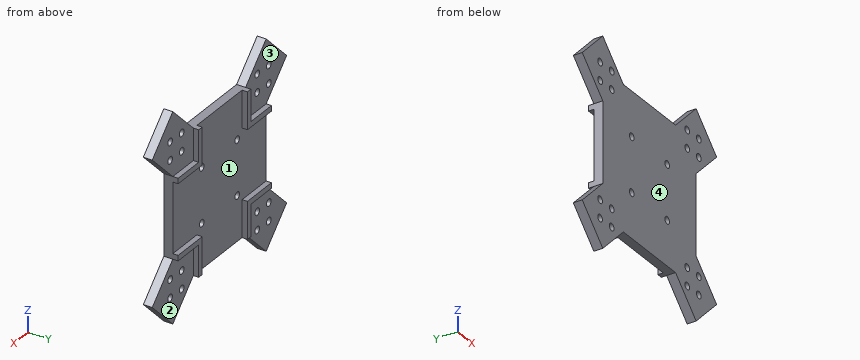
from build123d import *

# Parameters (mm, degrees)
EXTRUDE_1_DEPTH     = 5
EXTRUDE_2_DEPTH     = 3
SKETCH_4_R          = 2
CUT_EXTRUDE_1_DEPTH = 5
SKETCH_6_R          = 2
CUT_EXTRUDE_2_DEPTH = 5


with BuildPart() as part:
    # 스케치1 → 보스-돌출1 (new body)
    with BuildSketch(Plane(origin=(0, 0, 0), x_dir=(1, 0, 0), z_dir=(0, 1, 0))):
        Polygon((-40.17766953, 22.5), (-57.855339059, 40.17766953), (-40.17766953, 57.855339059), (-22.5, 40.17766953), align=None)
        Polygon((-22.5, 40.17766953), (22.5, -40.17766953), (-22.5, -40.17766953), (-40.17766953, -22.5), (-40.17766953, 22.5), align=None)
        Polygon((-40.17766953, -57.855339059), (-57.855339059, -40.17766953), (-40.17766953, -22.5), (-22.5, -40.17766953), align=None)
        Polygon((-22.5, 40.17766953), (22.5, 40.17766953), (40.17766953, 22.5), (40.17766953, -22.5), (22.5, -40.17766953), align=None)
        Polygon((40.17766953, -57.855339059), (22.5, -40.17766953), (40.17766953, -22.5), (57.855339059, -40.17766953), align=None)
        Polygon((40.17766953, 22.5), (22.5, 40.17766953), (40.17766953, 57.855339059), (57.855339059, 40.17766953), align=None)
    extrude(amount=EXTRUDE_1_DEPTH)

    # 스케치2 → 보스-돌출2 (add)
    with BuildSketch(Plane(origin=(0, 5, 0), x_dir=(1, 0, 0), z_dir=(0, 1, 0))):
        Polygon((-40.17766953, -19.5), (-40.17766953, -22.5), (-22.5, -22.5), (-22.5, -40.17766953), (-19.5, -40.17766953), (-19.5, -19.5), align=None)
        Polygon((-19.5, 40.17766953), (-22.5, 40.17766953), (-22.5, 22.5), (-40.17766953, 22.5), (-40.17766953, 19.5), (-19.5, 19.5), align=None)
        Polygon((40.17766953, 19.5), (40.17766953, 22.5), (22.5, 22.5), (22.5, 40.17766953), (19.5, 40.17766953), (19.5, 19.5), align=None)
        Polygon((19.5, -40.17766953), (22.5, -40.17766953), (22.5, -22.5), (40.17766953, -22.5), (40.17766953, -19.5), (19.5, -19.5), align=None)
    extrude(amount=EXTRUDE_2_DEPTH)

    # 스케치4 → 컷-돌출1 (cut)
    with BuildSketch(Plane(origin=(0, 0, 0), x_dir=(1, 0, 0), z_dir=(0, 1, 0))):
        with Locations(Location((-42.5, -42.5, 0), (0, 0, 270))):
            Circle(SKETCH_4_R)
        with Locations(Location((-32.5, -42.5, 0), (0, 0, 270))):
            Circle(SKETCH_4_R)
        with Locations(Location((-42.5, -32.5, 0), (0, 0, 270))):
            Circle(SKETCH_4_R)
        with Locations(Location((-32.5, -32.5, 0), (0, 0, 270))):
            Circle(SKETCH_4_R)
        with Locations(Location((-32.5, 32.5, 0), (0, 0, 270))):
            Circle(SKETCH_4_R)
        with Locations(Location((-42.5, 32.5, 0), (0, 0, 270))):
            Circle(SKETCH_4_R)
        with Locations(Location((-42.5, 42.5, 0), (0, 0, 270))):
            Circle(SKETCH_4_R)
        with Locations(Location((-32.5, 42.5, 0), (0, 0, 270))):
            Circle(SKETCH_4_R)
        with Locations(Location((32.5, 32.5, 0), (0, 0, 270))):
            Circle(SKETCH_4_R)
        with Locations(Location((32.5, 42.5, 0), (0, 0, 270))):
            Circle(SKETCH_4_R)
        with Locations(Location((42.5, 42.5, 0), (0, 0, 270))):
            Circle(SKETCH_4_R)
        with Locations(Location((42.5, 32.5, 0), (0, 0, 270))):
            Circle(SKETCH_4_R)
        with Locations(Location((32.5, -32.5, 0), (0, 0, 270))):
            Circle(SKETCH_4_R)
        with Locations(Location((42.5, -32.5, 0), (0, 0, 270))):
            Circle(SKETCH_4_R)
        with Locations(Location((42.5, -42.5, 0), (0, 0, 270))):
            Circle(SKETCH_4_R)
        with Locations(Location((32.5, -42.5, 0), (0, 0, 270))):
            Circle(SKETCH_4_R)
    extrude(amount=CUT_EXTRUDE_1_DEPTH, mode=Mode.SUBTRACT)

    # 스케치6 → 컷-돌출2 (cut)
    with BuildSketch(Plane(origin=(0, 0, 0), x_dir=(1, 0, 0), z_dir=(0, 1, 0))):
        with Locations(Location((-15.25, 15.25, 0), (0, 0, 270))):
            Circle(SKETCH_6_R)
        with Locations(Location((15.25, -15.25, 0), (0, 0, 270))):
            Circle(SKETCH_6_R)
        with Locations(Location((15.25, 15.25, 0), (0, 0, 270))):
            Circle(SKETCH_6_R)
        with Locations(Location((-15.25, -15.25, 0), (0, 0, 270))):
            Circle(SKETCH_6_R)
    extrude(amount=CUT_EXTRUDE_2_DEPTH, mode=Mode.SUBTRACT)


solid = part.part
Can you work these out from the model? Positions are in its coordinate system, mm. Face numbers are marked on the shaded views. A direction names the side the tool comes from. Round coordinates to 2 decimals unless told otherwise and drop trailing zeros. Order: outer loops, then holes, each group sorted by start corner. A loop starts at its lowest first (then second) coordinate and runs counter-clockwise, first axis right, second up. Notation, with made-up numbers: (40.5, 8) -> (62.5, 8) arc R30 cw to (62.5, 33) -> close; hole circle Ø3 at (10, -8.5). An arc over 180 degrees is marked (long way). Write each question's results on one line, items separated by ' | '. Start each with the question number.
Item 1: If we section it at D-D, the plane z = -48: Write out the boundary of the cut face in (x, y).
Item 2: If we section it at B-B, the plane x = 15.25: Write out the boundary of the cut face in (y, z).
Item 3: If we section it at A-A, the plane z = 15.25: Write out the boundary of the cut face in (x, y), then the cut area to 3 significant figures.
Item 4: Which directions (+Z, -Z, +X, -X, +Y, -Y) give clear straight access to the entire face, cutting with the end or side of a thin tool? Please do the marked faces 3 and 4.
Item 5: Please list where these lines run through material, in increasing order: L1, parallel to X at y = 2, z = 42.5; L2, parallel to X at y = 7.75, z = -36; L3, parallel to X at y = 0.75, z = 43.
Item 6: Will these pins go through, and if not, where does the flat tip stop? pin 1 (3.5 mm diameter, centred on y = 7, z = -27, fed in from +X); pin 2 (2.5 mm diameter, centred on x = 15.25, z = -15.25, fed in from -Y); pin 3 (1.5 mm diameter, centred on x = 28, y = 7, fed in from -Z); pin 4 (10 mm diameter, centred on x = 0.5, z = -31.5, fed in from +Y).
Item 7: Thinking about a two-plate mould opening in X: for the marked faces 1 and 2, which applies, +X half, -X half, draft (parallel to the pull), parting line (faces both ways), or undercut?
Item 8: If we section it at C-C, the plane x = 32.5: Write out the boundary of the cut face in (y, z), then the cut area to 3 significant figures.
Results:
1) outline: (-50.03, 0) -> (-30.32, 0) -> (-30.32, 5) -> (-50.03, 5) -> close; (30.32, 0) -> (50.03, 0) -> (50.03, 5) -> (30.32, 5) -> close
2) outline: (0, -40.18) -> (5, -40.18) -> (5, -17.25) -> (0, -17.25) -> close; (0, -13.25) -> (5, -13.25) -> (5, 13.25) -> (0, 13.25) -> close; (0, 17.25) -> (5, 17.25) -> (5, 40.18) -> (0, 40.18) -> close
3) outline: (-40.18, 0) -> (-17.25, 0) -> (-17.25, 5) -> (-40.18, 5) -> close; (-13.25, 0) -> (13.25, 0) -> (13.25, 5) -> (-13.25, 5) -> close; (17.25, 0) -> (40.18, 0) -> (40.18, 5) -> (17.25, 5) -> close | area: 362 mm2
4) face 3: +Z, -X, +Y | face 4: +Z, -Z, +X, -X, -Y
5) L1: x = -55.53 to -44.5, -40.5 to -34.5, -30.5 to -24.82, 24.82 to 30.5, 34.5 to 40.5, 44.5 to 55.53 | L2: x = -22.5 to -19.5, 19.5 to 22.5 | L3: x = -55.03 to -44.44, -40.56 to -34.44, -30.56 to -25.32, 25.32 to 30.56, 34.44 to 40.56, 44.44 to 55.03
6) pin 1: stops at x = 22.5 | pin 2: passes through | pin 3: stops at z = -22.5 | pin 4: stops at y = 5
7) face 1: undercut | face 2: draft
8) outline: (0, -50.18) -> (5, -50.18) -> (5, -44.5) -> (0, -44.5) -> close; (0, -40.5) -> (5, -40.5) -> (5, -34.5) -> (0, -34.5) -> close; (0, -30.5) -> (5, -30.5) -> (5, -22.5) -> (8, -22.5) -> (8, -19.5) -> (5, -19.5) -> (5, 19.5) -> (8, 19.5) -> (8, 22.5) -> (5, 22.5) -> (5, 30.5) -> (0, 30.5) -> close; (0, 34.5) -> (5, 34.5) -> (5, 40.5) -> (0, 40.5) -> close; (0, 44.5) -> (5, 44.5) -> (5, 50.18) -> (0, 50.18) -> close | area: 440 mm2
